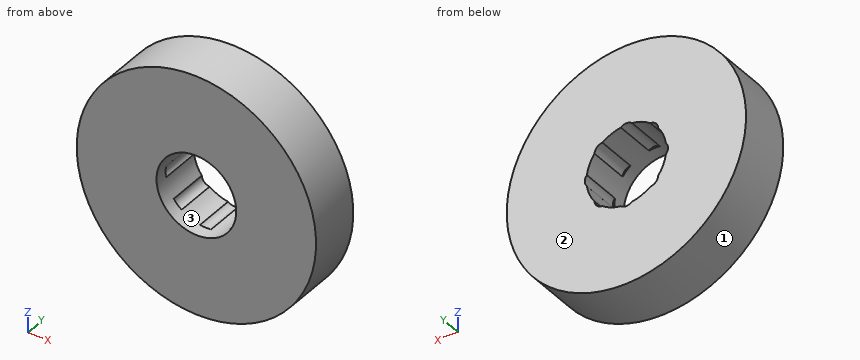
from build123d import *

# Parameters (mm, degrees)
SKETCH1_R           = 22.5
BOSS_EXTRUDE1_DEPTH = 10
SKETCH2_R           = 7.5
CUT_EXTRUDE1_DEPTH  = 34.35416016
SKETCH3_R           = 1.578036786
CUT_EXTRUDE2_DEPTH  = 7.540718
CIRPATTERN1_START   = 2.459282065
CIRPATTERN1_DEPTH   = 7.540717935


# Read off the part's stored shape, not the designer's step: CirPattern1
with BuildPart() as part:
    # Sketch1 → Boss-Extrude1 (new body)
    with BuildSketch(Plane(origin=(0, 0, 0), x_dir=(1, 0, 0), z_dir=(0, 1, 0))):
        with Locations(Location((0, 0, 0), (0, 0, 270))):
            Circle(SKETCH1_R)
    extrude(amount=BOSS_EXTRUDE1_DEPTH)

    # Sketch2 → Cut-Extrude1 (cut, through all)
    with BuildSketch(Plane(origin=(0, 0, 0), x_dir=(1, 0, 0), z_dir=(0, 1, 0))):
        with Locations(Location((0, 0, 0), (0, 0, 270))):
            Circle(SKETCH2_R)
    extrude(amount=CUT_EXTRUDE1_DEPTH, mode=Mode.SUBTRACT)

    # Sketch3 → Cut-Extrude2 (cut)
    with BuildSketch(Plane(origin=(0, 10, 0), x_dir=(1, 0, 0), z_dir=(0, 1, 0))):
        with Locations((-6.245323663, 0)):
            Circle(SKETCH3_R)
    extrude(amount=-CUT_EXTRUDE2_DEPTH, mode=Mode.SUBTRACT)

    # CirPattern1 outline → CirPattern1 (cut)
    with BuildSketch(Plane(origin=(0, 0, 0), x_dir=(1, 0, 0), z_dir=(0, 1, 0)).offset(CIRPATTERN1_START)):
        with BuildLine():
            ThreePointArc((-4.511638563, -5.991253414), (-5.303300859, -5.303300859), (-5.991253414, -4.511638563))
            ThreePointArc((-5.991253414, -4.511638563), (-5.531951226, -5.531951226), (-4.511638563, -5.991253414))
        make_face()
        with BuildLine():
            ThreePointArc((-4.511638563, 5.991253414), (-5.531951226, 5.531951226), (-5.991253414, 4.511638563))
            ThreePointArc((-5.991253414, 4.511638563), (-5.303300859, 5.303300859), (-4.511638563, 5.991253414))
        make_face()
        with BuildLine():
            ThreePointArc((1.046245695, -7.426666139), (0, -7.5), (-1.046245695, -7.426666139))
            ThreePointArc((-1.046245695, -7.426666139), (0, -7.82336045), (1.046245695, -7.426666139))
        make_face()
        with BuildLine():
            ThreePointArc((1.046245695, 7.426666139), (0, 7.82336045), (-1.046245695, 7.426666139))
            ThreePointArc((-1.046245695, 7.426666139), (0, 7.5), (1.046245695, 7.426666139))
        make_face()
        with BuildLine():
            ThreePointArc((5.991253414, -4.511638563), (5.303300859, -5.303300859), (4.511638563, -5.991253414))
            ThreePointArc((4.511638563, -5.991253414), (5.531951226, -5.531951226), (5.991253414, -4.511638563))
        make_face()
        with BuildLine():
            ThreePointArc((5.991253414, 4.511638563), (5.531951226, 5.531951226), (4.511638563, 5.991253414))
            ThreePointArc((4.511638563, 5.991253414), (5.303300859, 5.303300859), (5.991253414, 4.511638563))
        make_face()
        with BuildLine():
            ThreePointArc((7.426666139, 1.046245695), (7.5, 0), (7.426666139, -1.046245695))
            ThreePointArc((7.426666139, -1.046245695), (7.82336045, 0), (7.426666139, 1.046245695))
        make_face()
    extrude(amount=CIRPATTERN1_DEPTH, mode=Mode.SUBTRACT)


solid = part.part
The model under review builds one solid part; all positions refer to its coordinate system, in mm. Face numbers are marked on the shaded views. Coordinates: 2 decimals unless noted, no trailing zeros. Write each loop counter-clockwise with the first axis right and the second up, starting at its lowest first coordinate (ties: lowest second). Pieces come first, ordered by that corner, then holes. Notation, with made-up numbers: (24, 9) - (81, 9) arc R7 ccw to (81, 15) - close; hole circle Ø8 at (20, -15). An arc over 180 degrees is marked (long way). Answer as a JSON object with one key per item and string values. Group by question number.
1. Add section C-C (x = 2). Give the boundary of the cut face in (y, z).
2. Clearance check with flat-ended pins moving along their axes: pin 1 Ø2 at (x, y) = (5, 2) entering from -Z; pin 2 Ø5 at (y, z) = (3.5, -12.5) entering from +X; pin 3 Ø2 at (y, z) = (8, 3) entering from +X. State where each tip first meets the part, or that it passes through.
3. To check wall thickness, follow probe 1 along X at (y, z) = (8.25, 0); probe 2 along Z at (x, y) = (4.5, 3); probe 3 along X at (y, z) = (1.75, -5). State the ranges of each line that lie inside material, in increasing order.
4. Mouldability with a two-part tool opening along Z and no side actions: class the marked faces 1, 2 and 3 as pulls with the +Z half, pulls with the -Z half, needs draft (parallel to the pull), parting line crosses it, or undercut.
5. Add section B-B (y = 3). Give the boundary of the cut face in (x, z).
6. Add section D-D (x = 17). Give the boundary of the cut face in (y, z).
7. Add section A-A (z = 0). Give the boundary of the cut face in (x, y).
Findings:
{
 "1": {"outline": "(0, -22.41) - (10, -22.41) - (10, -7.23) - (0, -7.23) - close; (0, 7.23) - (10, 7.23) - (10, 22.41) - (0, 22.41) - close"},
 "2": {"pin 1": "z = -22.14", "pin 2": "x = 20.16", "pin 3": "x = 22.41"},
 "3": {"probe 1": "-22.5 to -7.82, 7.82 to 22.5", "probe 2": "-22.05 to -6, 6 to 22.05", "probe 3": "-21.94 to -5.59, 5.59 to 21.94"},
 "4": {"face 1": "parting line crosses it", "face 2": "needs draft", "face 3": "undercut"},
 "5": {"outline": "circle Ø45 at (0, 0); hole (-7.43, -1.05) arc R7.5 ccw to (-5.99, -4.51) arc R1.58 ccw to (-4.51, -5.99) arc R7.5 ccw to (-1.05, -7.43) arc R1.58 ccw to (1.05, -7.43) arc R7.5 ccw to (4.51, -5.99) arc R1.58 ccw to (5.99, -4.51) arc R7.5 ccw to (7.43, -1.05) arc R1.58 ccw to (7.43, 1.05) arc R7.5 ccw to (5.99, 4.51) arc R1.58 ccw to (4.51, 5.99) arc R7.5 ccw to (1.05, 7.43) arc R1.58 ccw to (-1.05, 7.43) arc R7.5 ccw to (-4.51, 5.99) arc R1.58 ccw to (-5.99, 4.51) arc R7.5 ccw to (-7.43, 1.05) arc R1.58 ccw to start"},
 "6": {"outline": "(0, -14.74) - (10, -14.74) - (10, 14.74) - (0, 14.74) - close"},
 "7": {"outline": "(-22.5, 0) - (-7.5, 0) - (-7.5, 2.46) - (-7.82, 2.46) - (-7.82, 10) - (-22.5, 10) - close; (7.5, 0) - (22.5, 0) - (22.5, 10) - (7.82, 10) - (7.82, 2.46) - (7.5, 2.46) - close"}
}
